```python
from build123d import *

# Parameters (mm, degrees)
SKETCH1_R           = 0.5
SKETCH1_R_2         = 1.575
SKETCH1_W           = 12
SKETCH1_H           = 4
BOSS_EXTRUDE1_DEPTH = 3


with BuildPart() as part:
    # Sketch1 → Boss-Extrude1 (new body)
    with BuildSketch(Plane(origin=(0, 0, 0), x_dir=(1, 0, 0), z_dir=(0, 1, 0))):
        with BuildLine():
            add(Edge.make_bspline(
                [(22.5, -16.5625), (34.262295129, -13.118708317), (45, -6.25)],
                knots=[0.479061635, 0.479061635, 0.479061635, 1, 1, 1], degree=2))
            ThreePointArc((45, -6.25), (47.588834765, 0), (45, 6.25))
            add(Edge.make_bspline(
                [(22.5, 16.5625), (34.262295129, 13.118708317), (45, 6.25)],
                knots=[0.479061635, 0.479061635, 0.479061635, 1, 1, 1], degree=2))
            Line((22.5, 16.5625), (0, 20))
            ThreePointArc((0, 20), (-20, 0), (0, -20))
            Line((0, -20), (22.5, -16.5625))
        make_face()
        with Locations(Location((0, -16.15, 0), (0, 0, 270))):
            Circle(SKETCH1_R, mode=Mode.SUBTRACT)
        with Locations(Location((0, -13.15, 0), (0, 0, 270))):
            Circle(SKETCH1_R, mode=Mode.SUBTRACT)
        with Locations(Location((0, -10.25, 0), (0, 0, 270))):
            Circle(SKETCH1_R_2, mode=Mode.SUBTRACT)
        with Locations(Location((-16.15, 0, 0), (0, 0, 270))):
            Circle(SKETCH1_R, mode=Mode.SUBTRACT)
        with BuildLine():
            ThreePointArc((-13.65, 0), (-13.15, 0.5), (-12.65, 0))
            ThreePointArc((-12.65, 0), (-13.15, -0.5), (-13.65, 0))
        make_face(mode=Mode.SUBTRACT)
        with BuildLine():
            ThreePointArc((-7.65, 0), (-7.15, 0.5), (-6.65, 0))
            ThreePointArc((-6.65, 0), (-7.15, -0.5), (-7.65, 0))
        make_face(mode=Mode.SUBTRACT)
        with Locations(Location((0, -7.15, 0), (0, 0, 270))):
            Circle(SKETCH1_R, mode=Mode.SUBTRACT)
        with BuildLine():
            ThreePointArc((3.177944539, 2.429129166), (1.282228888, -3.78891661), (-4, 0))
            ThreePointArc((-4, 0), (-1.282228888, 3.78891661), (3.177944539, 2.429129166))
        make_face(mode=Mode.SUBTRACT)
        with Locations(Location((7.15, 0, 0), (0, 0, 270))):
            Circle(SKETCH1_R, mode=Mode.SUBTRACT)
        with Locations(Location((10.25, 0, 0), (0, 0, 270))):
            Circle(SKETCH1_R_2, mode=Mode.SUBTRACT)
        with Locations(Location((13.15, 0, 0), (0, 0, 270))):
            Circle(SKETCH1_R, mode=Mode.SUBTRACT)
        with Locations(Location((16.15, 0, 0), (0, 0, 270))):
            Circle(SKETCH1_R, mode=Mode.SUBTRACT)
        with BuildLine():
            ThreePointArc((-11.825, 0), (-10.25, 1.575), (-8.675, 0))
            ThreePointArc((-8.675, 0), (-10.25, -1.575), (-11.825, 0))
        make_face(mode=Mode.SUBTRACT)
        with Locations(Location((0, 7.15, 0), (0, 0, 270))):
            Circle(SKETCH1_R, mode=Mode.SUBTRACT)
        with Locations(Location((0, 10.25, 0), (0, 0, 270))):
            Circle(SKETCH1_R_2, mode=Mode.SUBTRACT)
        with Locations(Location((0, 13.15, 0), (0, 0, 270))):
            Circle(SKETCH1_R, mode=Mode.SUBTRACT)
        with Locations(Location((0, 16.15, 0), (0, 0, 270))):
            Circle(SKETCH1_R, mode=Mode.SUBTRACT)
        with Locations((31.5, 0)):
            Rectangle(SKETCH1_W, SKETCH1_H, mode=Mode.SUBTRACT)
    extrude(amount=BOSS_EXTRUDE1_DEPTH)


solid = part.part
```
Geometry check sheet. Reference: the model listing, model coordinates, mm. A direction names the side the tool comes from. Round coordinates to 2 decimals unless told otherwise and drop trailing zeros. Loops run counter-clockwise (first coordinate to the right, second up) from the corner with the lowest first, then second, coordinate; pieces in that order, holes last. Notation, with made-up numbers: M -20,-1 L 8,-1 A21 cw 8,21 Z; hole C 17,81 d6. An arc over 180 degrees is marked long. Return JSON: item names as keys, results as strings. Group by question number.
(1) Section check A-A, the plane x = -10.25. Enter the section's corners in (y, z) (3 decimals), and give its area (3 significant figures).
(2) Set-up check for faces 1 (the face through (37.5, 1, 0)), 2 (the face through (6, 3, 0)): record each of +Z, -Z, +X, -X, +Y, -Y from which the full face is reachable in a straight line by a thin tool's end or side.
(3) Go/stop test with flat-tipped pins: pin 1 (7 mm diameter, centred on x = 0, z = 0, fed in from -Y); pin 2 (1 mm diameter, centred on x = 8.5, z = 6, fed in from -Y); pin 3 (1.5 mm diameter, centred on y = 1, z = 0, fed in from -X). Record where each tip stops, or that it passes through.
(4) Mould release check, pull along Z, two halves, no side actions. Record for faces 3 (the face through (6, 0, 0)), 4 (the face through (-0.96, 1.48, 9)), 5 (the face through (11.092, 1.479, 18.305)), 6 (the face through (11.407, 1.479, -18.257)): pulls with the +Z half, pulls with the -Z half, needs draft (parallel to the pull), parting line crosses it, or undercut.
(5) Scan lines: line 1 along Z through (x, y) = (31, 1.5); line 2 along Z through (x, y) = (11.5, 2.8); line 3 along X through (y, z) = (1.8, -10.5). Record each from-to range of solid material in increasing order. Write a range as [from, to].
(6) Section check C-C, the plane x = 17.5. Enter the section's corners in (y, z), and give its area (3 significant figures).
(7) Section check B-B, the plane y = 1.15. Give the number of separate pieces and of enclosed holes in the cut face, and give its area (3 significant figures).
Data:
{
 "1": {"outline": "M 0,-17.174 L 3,-17.174 L 3,-1.575 L 0,-1.575 Z; M 0,1.575 L 3,1.575 L 3,17.174 L 0,17.174 Z", "area": "93.6 mm²"},
 "2": {"face 1": "+Y, -Y", "face 2": "+Z, -Z, +X, -X, +Y"},
 "3": {"pin 1": "through", "pin 2": "y = 0", "pin 3": "x = -20"},
 "4": {"face 3": "needs draft", "face 4": "undercut", "face 5": "pulls with the +Z half", "face 6": "pulls with the -Z half"},
 "5": {"line 1": "[-13.57, -2], [2, 13.57]", "line 2": "[-18.24, -0.96], [0.96, 18.24]", "line 3": "[-17.02, -1.56], [1.56, 37.63]"},
 "6": {"outline": "M 0,-17.33 L 3,-17.33 L 3,17.33 L 0,17.33 Z", "area": "104 mm²"},
 "7": {"separate pieces": "1", "enclosed holes": "18", "area": "1,880 mm²"}
}
